Verification items for the finished model (mm, model axes). A direction names the side the tool comes from. Give positions to 0.01 mm unless a question says otherwise; leave off trailing zeros. Write each loop counter-clockwise with the first axis right and the second up, starting at its lowest first coordinate (ties: lowest second). Pieces come first, ordered by that corner, then holes. Notation, with made-up numbers: M 35.25,11 L 82.25,11 A23 ccw 82.25,22 Z; hole C -38,35.25 d4. An arc over 180 degrees is marked long. Answer as a JSON object with one key per item and string values.
```python
from build123d import *

# Parameters (mm, degrees)
F0_R          = 11.25
F1_DEPTH      = 15
F1_DEPTH_BACK = 15
F4_DEPTH      = 30.001
F2_R          = 8.75
F5_DEPTH      = 11
F3_R          = 8.75
F6_DEPTH      = 11
F8_D          = 5
F9_R          = 2
F10_R         = 2


with BuildPart() as f1:
    # F0 (on Top) → F1 (new body, two sides)
    with BuildSketch(Plane.XY) as f1_sk:
        Circle(F0_R)
    extrude(amount=F1_DEPTH)
    extrude(f1_sk.sketch, amount=-F1_DEPTH_BACK)

    # F2 (on face) → F4 (cut, through all)
    with BuildSketch(Plane.XY.offset(15)):
        with BuildLine():
            Line((6.4527349089, -9.2154604983), (-6.4527349089, -9.2154604983))
            ThreePointArc((-6.4527349089, -9.2154604983), (0, -11.25), (6.4527349089, -9.2154604983))
        make_face()
    extrude(amount=-F4_DEPTH, mode=Mode.SUBTRACT)

    # F2 (on face) → F5 (cut)
    with BuildSketch(Plane.XY.offset(15)):
        Circle(F2_R)
    extrude(amount=-F5_DEPTH, mode=Mode.SUBTRACT)

    # F3 (on face) → F6 (cut)
    with BuildSketch(Plane(origin=(0, 0, -15), x_dir=(1, 0, 0), z_dir=(0, 0, -1))):
        Circle(F3_R)
    extrude(amount=-F6_DEPTH, mode=Mode.SUBTRACT)

    # F8 (through all)
    with Locations(Plane.XZ.offset(9.2154604983)):
        with Locations((0, 0)):
            Hole(F8_D / 2)

    # F9
    f9_edges = [f1.edges().sort_by_distance(p)[0] for p in [
        (-8.75, 0, 4),
    ]]
    fillet(f9_edges, radius=F9_R)

    # F10
    f10_edges = [f1.edges().sort_by_distance(p)[0] for p in [
        (-8.75, 0, -4),
    ]]
    fillet(f10_edges, radius=F10_R)


solid = f1.part
```
1) Access from +Z, -Z, +X, -X, +Y, -Y to the whole of each face (thin tool, end or side, straight path). Record for faces 1 (the face through (0.54, 1.16, -2.44)), 2 (the face through (0, 0, 4)), 3 (the face through (0, 0, -4)).
Completed:
{"face 1": "+Y, -Y", "face 2": "+Z", "face 3": "-Z"}
2) Thickness scan on L1, parallel to Y at x = 0, z = -10.75; L2, parallel to X at y = 0, z = -12.75; L3, parallel to Z at x = 0, y = -0.75. Record the ranges inside material, lowest first.
Completed:
{"L1": "y = -9.22 to -8.75, 8.75 to 11.25", "L2": "x = -11.25 to -8.75, 8.75 to 11.25", "L3": "z = -4 to -2.5, 2.5 to 4"}
3) Section check A-A on y = 0. Record the boundary of the cut face in (x, z), and give its area (3 significant figures).
Completed:
{"outline": "M -11.25,-15 L -8.75,-15 L -8.75,-6 A2 cw -6.75,-4 L 6.75,-4 A2 cw 8.75,-6 L 8.75,-15 L 11.25,-15 L 11.25,15 L 8.75,15 L 8.75,6 A2 cw 6.75,4 L -6.75,4 A2 cw -8.75,6 L -8.75,15 L -11.25,15 Z; hole C 0,0 d5", "area": "274 mm2"}
4) Section check B-B on x = 0. Record the boundary of the cut face in (y, z), and give its area (3 significant figures).
Completed:
{"outline": "M -9.22,-15 L -8.75,-15 L -8.75,-6 A2 cw -6.75,-4 L 6.75,-4 A2 cw 8.75,-6 L 8.75,-15 L 11.25,-15 L 11.25,-2.5 L -9.22,-2.5 Z; M -9.22,2.5 L 11.25,2.5 L 11.25,15 L 8.75,15 L 8.75,6 A2 cw 6.75,4 L -6.75,4 A2 cw -8.75,6 L -8.75,15 L -9.22,15 Z", "area": "130 mm2"}
5) Section check C-C on z = 0. Record the boundary of the cut face in (x, y), and give its area (3 significant figures).
Completed:
{"outline": "M -6.45,-9.22 L -2.5,-9.22 L -2.5,10.97 A11.25 ccw Z; M 2.5,-9.22 L 6.45,-9.22 A11.25 ccw 2.5,10.97 Z", "area": "278 mm2"}
6) Go/stop test with flat-tipped pins: pin 1 (2 mm diameter, centred on y = -5, z = -3, fed in from -X); pin 2 (4 mm diameter, centred on x = -8.5, z = 11.5, fed in from +Y); pin 3 (1 mm diameter, centred on y = 7, z = -5, fed in from +X). Record where each tip stops, or that it passes through.
Completed:
{"pin 1": "stops at x = -10.51", "pin 2": "stops at y = 9.18", "pin 3": "stops at x = 9.18"}
7) Section check D-D on z = -7. Record the boundary of the cut face in (x, y), and give its area (3 significant figures).
Completed:
{"outline": "M -6.45,-9.22 L 6.45,-9.22 A11.25 ccw long Z; hole C 0,0 d17.5", "area": "139 mm2"}
8) Release check for a two-part mould opening along Y. For faces 4 (the face through (-5.7, 9.7, 0.2)), 5 (the face through (-6.944, 5.324, -10.563)), 6 (the face through (-4, 8, -15)) record: pulls with the +Y half, pulls with the -Y half, needs draft (parallel to the pull), parting line crosses it, or undercut.
Completed:
{"face 4": "parting line crosses it", "face 5": "undercut", "face 6": "needs draft"}
